Input: part model. Units: mm. Frame: model coordinates. Face numbers are marked on the shaded views. A direction names the side the tool comes from. Coordinates: 2 decimals unless noted, no trailing zeros. Write each loop counter-clockwise with the first axis right and the second up, starting at its lowest first coordinate (ties: lowest second). Pieces come first, ordered by that corner, then holes. Notation, with made-up numbers: M -11,17.25 L 23,17.25 A19 cw 23,22.25 Z; hole C -7,-10.5 d2. An arc over 180 degrees is marked long. Use one line per item in the form item = value.
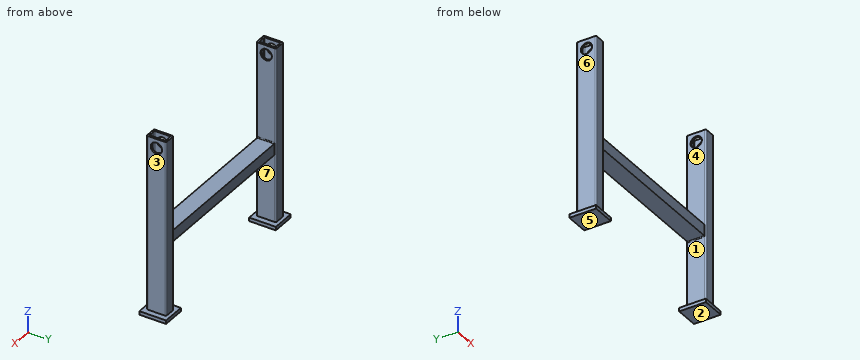
from build123d import *

# Parameters (mm, degrees)
F0_W        = 130
F0_H        = 150
F1_DEPTH    = 20
F2_W        = 65
F2_H        = 110
F2_W_2      = 45
F2_H_2      = 90
F3_DEPTH    = 980
F4_R        = 7
F5_R        = 5.08
F6_W        = 96
F6_H        = 63.5
F6_W_2      = 73.66
F6_H_2      = 45.72
F7_DEPTH    = 450
F8_T1_DEPTH = 96
F9_T1_DEPTH = 96
F13_D       = 63.5


# Not quite as in the source:
# - a fillet or chamfer that OpenCascade refuses, or shapes differently, is made with other operations: its cross-section is extruded or revolved along the edge and cut away or added


with BuildPart() as f1:
    # F0 (on Top) → F1 (new body)
    with BuildSketch(Plane.XY):
        with Locations((515, 0)):
            Rectangle(F0_W, F0_H)
    extrude(amount=F1_DEPTH)

    # F2 (on face) → F3 (join)
    with BuildSketch(Plane.XY.offset(20)):
        with Locations((515, 0)):
            Rectangle(F2_W, F2_H)
        with Locations((515, 0)):
            Rectangle(F2_W_2, F2_H_2, mode=Mode.SUBTRACT)
    extrude(amount=F3_DEPTH)

    # F4
    f4_edges = [f1.edges().sort_by_distance(p)[0] for p in [
        (547.5, -55, 510),
        (482.5, -55, 510),
        (547.5, 55, 510),
        (482.5, 55, 510),
    ]]
    fillet(f4_edges, radius=F4_R)

    # F5
    f5_edges = [f1.edges().sort_by_distance(p)[0] for p in [
        (492.5, 45, 510),
        (492.5, -45, 510),
        (537.5, -45, 510),
        (537.5, 45, 510),
    ]]
    fillet(f5_edges, radius=F5_R)

    # F6 (on face) → F7 (join)
    with BuildSketch(Plane(origin=(482.5, 0, 0), x_dir=(0, -1, 0), z_dir=(-1, 0, 0))):
        with Locations((0, 431.75)):
            Rectangle(F6_W, F6_H)
        with Locations((0.26, 431.75)):
            Rectangle(F6_W_2, F6_H_2, mode=Mode.SUBTRACT)
    extrude(amount=F7_DEPTH)

    # F8: fillet of radius 5 on 1 edges, made by hand

    # F8_s2 → F8_t1 (join)
    with BuildSketch(Plane.XZ.offset(-48)):
        with BuildLine():
            ThreePointArc((482.5, 468.5), (481.0355339059, 464.9644660941), (477.5, 463.5))
            Line((477.5, 463.5), (482.5, 463.5))
            Line((482.5, 463.5), (482.5, 468.5))
        make_face()
    extrude(amount=F8_T1_DEPTH)

    # F9: fillet of radius 5 on 1 edges, made by hand

    # F9_s2 → F9_t1 (join)
    with BuildSketch(Plane.XZ.offset(-48)):
        with BuildLine():
            ThreePointArc((482.5, 395), (481.0355339059, 398.5355339059), (477.5, 400))
            Line((477.5, 400), (482.5, 400))
            Line((482.5, 400), (482.5, 395))
        make_face()
    extrude(amount=F9_T1_DEPTH)

    # F11: F1 across face


with BuildPart() as f1_1:
    add(f1.part)
    add(f1.part.mirror(Plane(origin=(32.5, 0, 0), x_dir=(0, -1, 0), z_dir=(-1, 0, 0))))

    # F13 (through all)
    with Locations(Plane.YZ.offset(547.5)):
        with Locations((0, 947.7953910828)):
            Hole(F13_D / 2)


solid = f1_1.part
(1) Line query: probe 1 along X at (y, z) = (-16, 386.5); probe 2 along X at (y, z) = (21, 408); probe 3 along Z at (x, y) = (-423.25, 0). Output: solid intervals per line, ascending.
Computed:
probe_1 = -482.5 to -472.5, -427.5 to -417.5, 482.5 to 492.5, 537.5 to 547.5
probe_2 = -482.5 to -472.5, -427.5 to 492.5, 537.5 to 547.5
probe_3 = 0 to 916.05, 979.55 to 1000
(2) Pull-direction query (X, two-part tool) for the marked faces 5, 6 and 7; classes: pulls with the +X half, pulls with the -X half, needs draft (parallel to the pull), parting line crosses it, or undercut.
Computed:
face_5 = needs draft
face_6 = pulls with the -X half
face_7 = undercut
(3) Section query C-C on x = -259. Return the cut outline in (y, z).
Computed:
outline = M -48,400 L 48,400 L 48,463.5 L -48,463.5 Z; hole M -37.09,408.89 L 36.57,408.89 L 36.57,454.61 L -37.09,454.61 Z
(4) Section query D-D on x = -446. Return the cut outline in (y, z).
Computed:
outline = M -75,0 L 75,0 L 75,20 L 55,20 L 55,1000 L 45,1000 L 45,20 L -45,20 L -45,1000 L -55,1000 L -55,20 L -75,20 Z
(5) First-contact query: pin 1 Ø15.5 at (x, z) = (505.5, 578) entering from -Y; pin 2 Ø12 at (x, y) = (-162, 22) entering from +Z; pin 3 Ø13.5 at (x, y) = (522, 17.5) entering from +Z; pin 4 Ø12 at (x, y) = (-298.5, -56) entering from -Z. Flat tips, straight axial feed; report the tip coordinate or a pass-through.
Computed:
pin_1 = -55
pin_2 = 463.5
pin_3 = 20
pin_4 = through
(6) Set-up query: the marked faces 1, 2, 3 and 4. Return all of +Z, -Z, +X, -X, +Y, -Y with unobstructed straight access to the full face (end or side cutting, diameter ignored); none if empty.
Computed:
face_1 = +Y, -Y
face_2 = -Z, +X, -X, +Y, -Y
face_3 = +Z, +X, +Y, -Y
face_4 = +Z, +Y, -Y
(7) Section query A-A on z = 654.5. State how many separate pieces and enclosed holes the cut face has, plus the area to 3 significant figures.
Computed:
separate_pieces = 2
enclosed_holes = 2
area = 6,160 mm^2
